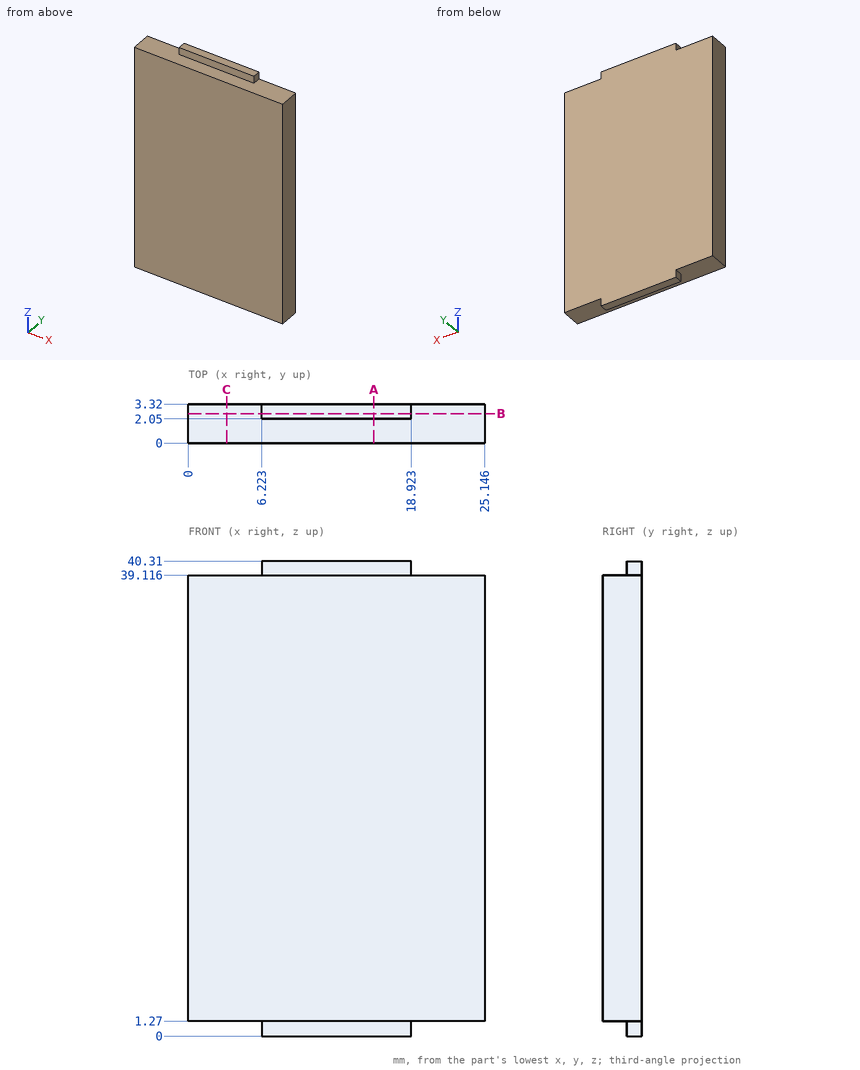
Input: dimensioned drawing with shaded views. Units: mm. Origin: part minimum x, y, z. Coordinates: 2 decimals unless noted, no trailing zeros. Order: outer loops, then holes, each group sorted by start corner. A loop starts at its lowest first (then second) coordinate and runs counter-clockwise, first axis right, second up. Notation, with made-up numbers: (-6.5, 2.25) - (51.5, 2.25) arc R23 ccw to (51.5, 27.25) - close; hole circle Ø3 at (60, 15). An arc over 180 degrees is marked (long way). Return JSON: item names as keys, results as strings. Group by question number.
1. Pin query (flat end, axial travel): pin 1 (0.6 mm diameter, centred on y = 2.5, z = 39.5, fed in from -X); pin 2 (0.6 mm diameter, centred on x = 11, z = 0.5, fed in from -Y); pin 3 (0.6 mm diameter, centred on y = 2.5, z = 0.5, fed in from +X). Return the tip coordinate at first contact, or that it passes through.
2. Cut plane A-A (x = 15.75). Output: boundary loops of the cut face in (y, z), plus the area to 3 significant figures.
3. Cut plane C-C (x = 3.25). Output: boundary loops of the cut face in (y, z), plus the area to 3 significant figures.
4. Cut plane B-B (y = 2.5). Output: boundary loops of the cut face in (x, z).
5. Material intervals for line 1 along Z through (x, y) = (1, 2.1), sorted ascending. Write a range as [from, to].
Resolved:
{
 "1": {"pin 1": "stops at x = 6.22", "pin 2": "stops at y = 2.05", "pin 3": "stops at x = 18.92"},
 "2": {"outline": "(0, 1.27) - (2.05, 1.27) - (2.05, 0) - (3.32, 0) - (3.32, 40.31) - (2.05, 40.31) - (2.05, 39.12) - (0, 39.12) - close", "area": "129 mm²"},
 "3": {"outline": "(0, 1.27) - (3.32, 1.27) - (3.32, 39.12) - (0, 39.12) - close", "area": "126 mm²"},
 "4": {"outline": "(0, 1.27) - (6.22, 1.27) - (6.22, 0) - (18.92, 0) - (18.92, 1.27) - (25.15, 1.27) - (25.15, 39.12) - (18.92, 39.12) - (18.92, 40.31) - (6.22, 40.31) - (6.22, 39.12) - (0, 39.12) - close"},
 "5": {"line 1": "z = [1.27, 39.12]"}
}
